CAD build for the part. Positions are in the model's coordinates, mm. Round coordinates to 2 decimals unless told otherwise and drop trailing zeros. Loops run counter-clockwise (first coordinate to the right, second up) from the corner with the lowest first, then second, coordinate; pieces in that order, holes last.
Autodesk Inventor part; units mm, degrees
ref_plane "YZ Plane" through (0, 0, 0) normal (1, 0, 0) x (0, 1, 0)
ref_plane "XZ Plane" through (0, 0, 0) normal (0, 1, 0) x (-1, 0, 0)
ref_plane "XY Plane" through (0, 0, 0) normal (0, 0, 1) x (1, 0, 0)
sketch "Sketch1" plane through (0, 0, 0) normal (1, 0, 0) x (0, 1, 0)
  circle A0 centre (0, 0) radius 2.921
  dimension "d0" = 5.842
extrude "Extrusion1" add sketch "Sketch1" along normal blind 152.4
sketch "Sketch2" plane through (152.4, 0, 0) normal (1, 0, 0) x (0, 0, -1)
  line L0 (-6.35, 6.35) -> (6.35, 6.35)
  line L1 (6.35, 6.35) -> (6.35, -6.35)
  line L2 (6.35, -6.35) -> (-6.35, -6.35)
  line L3 (-6.35, -6.35) -> (-6.35, 6.35)
  point P0 (0, 0)
  dimension "d5" = 12.7
  dimension "d6" = 12.7
  dimension "d7" = 6.35
  dimension "d8" = 6.35
extrude "Extrusion2" add sketch "Sketch2" along normal blind 34.417
sketch "Sketch3" plane through (152.4, -6.35, 6.35) normal (0, 0, 1) x (1, 0, 0)
  circle A0 centre (19.812, 6.35) radius 3.175
  line L0 (34.417, 12.7) -> (34.417, 0)
  point P0 (-152.4, 6.35)
  dimension "d12" = 0
  dimension "d9" = 6.35
  dimension "d10" = 14.605
extrude "Extrusion3" cut sketch "Sketch3" against normal blind 34.417
properties part number "SolenoidArm"
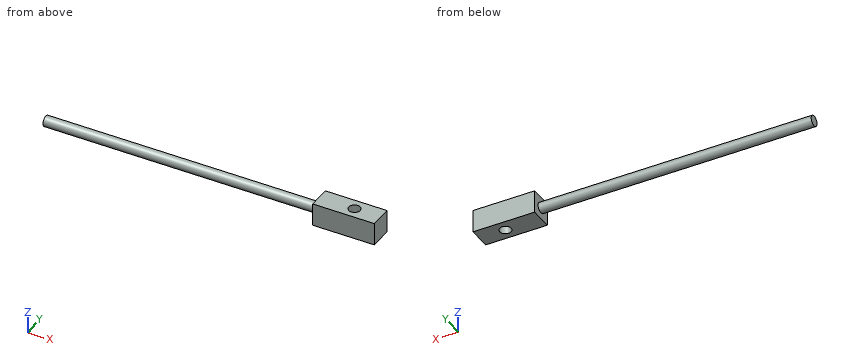
Item 1: Flat gauge pins, fed straight in: P1, Ø3, axis at y = -4, z = 2, coming from the -X side; P2, Ø1.5, axis at x = 83.5, y = -2, coming from the +Z side; P3, Ø3, axis at x = 115, y = 0, coming from the +Z side. Where does each tip first touch, or does it go through?
Answers follow:
P1: stops at x = 152.4
P2: stops at z = 2.64
P3: stops at z = 2.92
Item 2: Cut at C-C, the plane x = 62. Give the cut face in (y, z).
Answers follow:
outline: circle Ø5.84 at (0, 0)
Item 3: Cut at B-B, the plane z = 0. Give the cut face in (x, y) (3 decimals), plus the area to 3 significant figures.
Answers follow:
outline: (0, -2.921) - (152.4, -2.921) - (152.4, -6.35) - (186.817, -6.35) - (186.817, 6.35) - (152.4, 6.35) - (152.4, 2.921) - (0, 2.921) - close; hole circle Ø6.35 at (172.212, 0)
area: 1,300 mm2
Item 4: Cut at A-A, the plane y = 0. Give the cut face in (x, z).
Answers follow:
outline: (0, -2.92) - (152.4, -2.92) - (152.4, -6.35) - (169.04, -6.35) - (169.04, 6.35) - (152.4, 6.35) - (152.4, 2.92) - (0, 2.92) - close; (175.39, -6.35) - (186.82, -6.35) - (186.82, 6.35) - (175.39, 6.35) - close
Item 5: Probe line 1 (X direction, y = 4.25, z = -3.75); line 2 (X direction, y = 1.5, z = -4.5); line 3 (Z direction, x = 150, y = -0.25). List the from-to ranges inside material, lowest first.
Answers follow:
line 1: x = 152.4 to 186.82
line 2: x = 152.4 to 169.41, 175.01 to 186.82
line 3: z = -2.91 to 2.91
